For this review, take the finished solid that the model builds, in its own axes (mm). A direction names the side the tool comes from. Round coordinates to 2 decimals unless told otherwise and drop trailing zeros. Order: outer loops, then holes, each group sorted by start corner. A loop starts at its lowest first (then second) coordinate and runs counter-clockwise, first axis right, second up. Notation, with made-up numbers: M 33.25,1 L 56.25,1 A9 ccw 56.25,8 Z; hole C 82.25,47 d4. An arc over 180 degrees is marked long. Answer in a Markdown table with one row per item. Add a question column.
```python
from build123d import *

# Parameters (mm, degrees)
F0_W     = 228.6
F0_H     = 609.6
F1_DEPTH = 25.4
F2_W     = 431.8
F2_H     = 812.8
F3_DEPTH = 317.5
F4_R     = 3.175
F5_DEPTH = 25.4


with BuildPart() as f1:
    # F0 (on Top) → F1 (new body)
    with BuildSketch(Plane.XY):
        Rectangle(F0_W, F0_H)
    extrude(amount=F1_DEPTH)

    # F2 (on face) → F3 (join)
    with BuildSketch(Plane.XY.offset(25.4)):
        with Locations((-88.9, -107.95)):
            Rectangle(F2_W, F2_H)
    extrude(amount=F3_DEPTH)

    # F4 (on face) → F5 (cut)
    with BuildSketch(Plane(origin=(0, 0, 0), x_dir=(1, 0, 0), z_dir=(0, 0, -1))):
        with Locations((-50.8, -228.6)):
            Circle(F4_R)
        with Locations((19.05, -228.6)):
            Circle(F4_R)
        with Locations((-50.8, 146.05)):
            Circle(F4_R)
        with Locations((19.05, 146.05)):
            Circle(F4_R)
    extrude(amount=-F5_DEPTH, mode=Mode.SUBTRACT)


solid = f1.part
```
1. To check wall thickness, follow probe 1 along X at (y, z) = (228, 6); probe 2 along Y at (x, z) = (-50.8, 5) (3 decimals); probe 3 along X at (y, z) = (-146, 13). State the ranges of each line that lie inside material, in increasing order. Write a range as [from, to].
2. Consider section B-B on x = 82.5. Write out the cut boundary in (y, z), plus the area to 3 significant figures.
3. Consider section A-A on y = 55. Write out the cut boundary in (x, z).
4. Consider section D-D on y = -392. Write out the cut boundary in (x, z).
5. Consider section C-C on x = -253. Write out the cut boundary in (y, z), plus the area to 3 significant figures.
6. For faces 1 (the flat face through (-92, 298.45, 182)), 2 (the flat face through (114.3, -4, 13)), 3 (the flat face through (-114.3, -4, 13)), 4 (the flat face through (-2, -304.8, 13)), list the 3-axis set-ups (+Z, -Z, +X, -X, +Y, -Y) from which the entire face can be reached by the end or side of a thin tool; tool diameter is ignored.
7. Clearance check with flat-ended pins moving along their axes: pin 1 Ø1.9 at (x, y) = (-51.5, -145) entering from -Z; pin 2 Ø4 at (x, z) = (48.5, 247) entering from +Y; pin 3 Ø7.5 at (x, z) = (-16.5, 15) entering from -Y. State where each tip first meets the part, or that it passes through.
Solved:
| question | item | result |
|---|---|---|
| 1 | probe 1 | x = [-114.3, -53.92], [-47.68, 15.93], [22.17, 114.3] |
| 1 | probe 2 | y = [-304.8, -149.225], [-142.875, 225.425], [231.775, 304.8] |
| 1 | probe 3 | x = [-114.3, -53.97], [-47.63, 15.88], [22.22, 114.3] |
| 2 | outline | M -514.35,25.4 L -304.8,25.4 L -304.8,0 L 304.8,0 L 304.8,25.4 L 298.45,25.4 L 298.45,342.9 L -514.35,342.9 Z |
| 2 | area | 274,000 mm^2 |
| 3 | outline | M -304.8,25.4 L -114.3,25.4 L -114.3,0 L 114.3,0 L 114.3,25.4 L 127,25.4 L 127,342.9 L -304.8,342.9 Z |
| 4 | outline | M -304.8,25.4 L 127,25.4 L 127,342.9 L -304.8,342.9 Z |
| 5 | outline | M -514.35,25.4 L 298.45,25.4 L 298.45,342.9 L -514.35,342.9 Z |
| 5 | area | 258,000 mm^2 |
| 6 | face 1 | +Z, +X, -X, +Y |
| 6 | face 2 | -Z, +X, +Y, -Y |
| 6 | face 3 | -Z, -X, +Y, -Y |
| 6 | face 4 | -Z, +X, -X, -Y |
| 7 | pin 1 | stops at z = 25.4 |
| 7 | pin 2 | stops at y = 298.45 |
| 7 | pin 3 | stops at y = -304.8 |
